Can you work these out from the drawing? Everything is in mm from the part's minimum corner. A direction names the side the tool comes from. Give positions to 0.01 mm unless a question says otherwise; leave off trailing zeros. Write each loop counter-clockwise with the first axis right and the second up, starting at its lowest first coordinate (ties: lowest second). Pieces come first, ordered by that corner, then holes. Notation, with made-up numbers: (66.5, -34.5) -> (104.5, -34.5) arc R6 ccw to (104.5, -27.5) -> close; hole circle Ø2 at (8, 39). An arc over 180 degrees is marked (long way). Use one line per item in the form item = value.
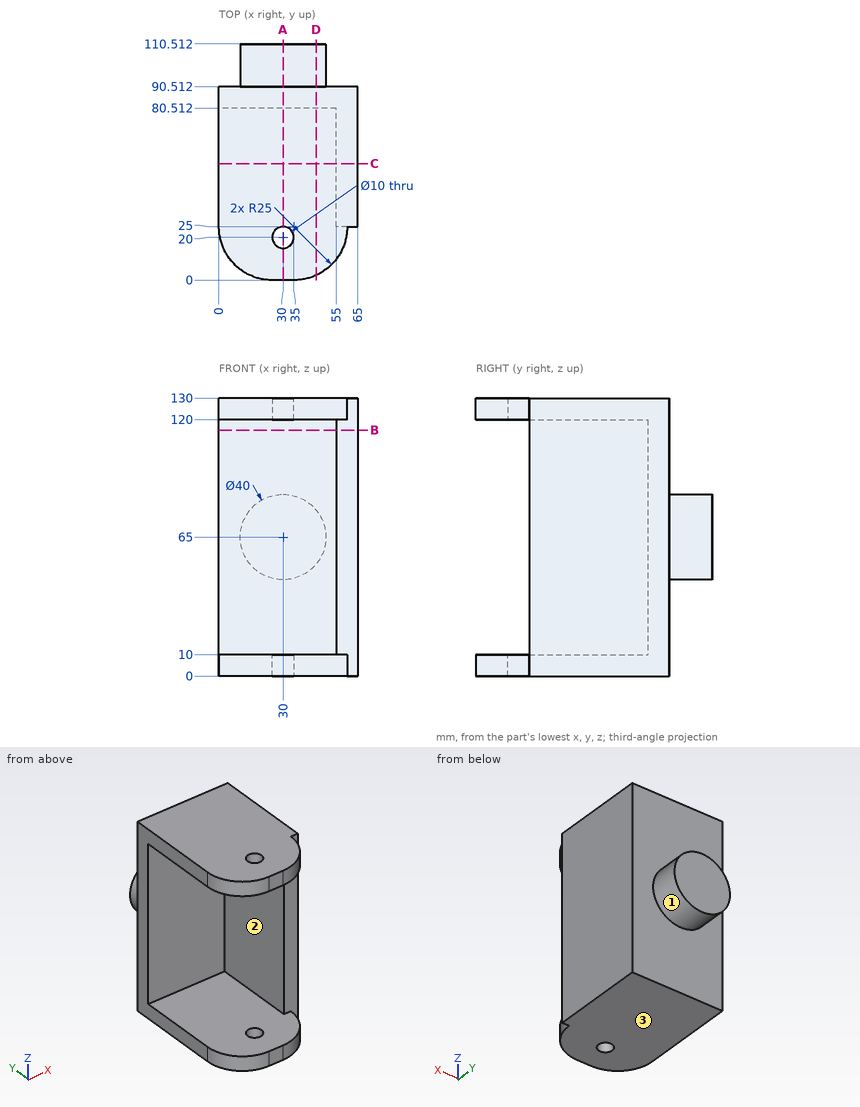
Q1. If I drill on line 1 along Z through (x, y) = (46.5, 17); line 2 along Y through (x, z) = (30, 125); line 3 along Y through (x, z) = (26, 90.5), over which ranges is the centre line in solid material (lowest first)? Write a range as from..to.
Result set:
line_1 = 0..10, 120..130
line_2 = 0..15, 25..90.51
line_3 = 80.51..90.51
Q2. Will these pins go through, and if not, where does the flat tip stop? pin 1 Ø6 at (x, z) = (24.5, 43) entering from -Y; pin 2 Ø8 at (x, z) = (62.5, 84) entering from -Y; pin 3 Ø5 at (y, z) = (58.5, 106.5) entering from -X; pin 4 Ø6 at (x, y) = (30, 20) entering from +Z.
Result set:
pin_1 = 80.51
pin_2 = 25
pin_3 = 55
pin_4 = through
Q3. I want a section at D-D, the plane x = 45.5. Write out the boundary of the cut face in (y, z), and give its area (3 significant figures).
Result set:
outline = (2.31, 0) -> (90.51, 0) -> (90.51, 52.36) -> (110.51, 52.36) -> (110.51, 77.64) -> (90.51, 77.64) -> (90.51, 130) -> (2.31, 130) -> (2.31, 120) -> (80.51, 120) -> (80.51, 10) -> (2.31, 10) -> close
area = 3,370 mm2
Q4. I want a section at B-B, the plane z = 115. Write out the boundary of the cut face in (x, y).
Result set:
outline = (0, 80.51) -> (55, 80.51) -> (55, 25) -> (65, 25) -> (65, 90.51) -> (0, 90.51) -> close
Q5. I want a section at A-A, the plane x = 30. Write out the boundary of the cut face in (y, z).
Result set:
outline = (0, 0) -> (15, 0) -> (15, 10) -> (0, 10) -> close; (0, 120) -> (15, 120) -> (15, 130) -> (0, 130) -> close; (25, 0) -> (90.51, 0) -> (90.51, 45) -> (110.51, 45) -> (110.51, 85) -> (90.51, 85) -> (90.51, 130) -> (25, 130) -> (25, 120) -> (80.51, 120) -> (80.51, 10) -> (25, 10) -> close
Q6. I want a section at C-C, the plane y = 54.5. Write out the boundary of the cut face in (x, z), and give its area (3 significant figures).
Result set:
outline = (0, 0) -> (65, 0) -> (65, 130) -> (0, 130) -> (0, 120) -> (55, 120) -> (55, 10) -> (0, 10) -> close
area = 2,400 mm2
Q7. Which directions (+Z, -Z, +X, -X, +Y, -Y) give clear straight access to the entire face, cutting with the end or side of a thin tool? Please do the marked faces 1, 2 and 3.
Result set:
face_1 = +Y
face_2 = -X, -Y
face_3 = -Z, +X, -X, +Y, -Y
